Could you check a few things on this model? Use its own coordinates, in mm. Face numbers are marked on the shaded views. A direction names the side the tool comes from. Give positions to 0.01 mm unless a question says otherwise; leave off trailing zeros. Write each loop counter-clockwise with the first axis right and the second up, starting at its lowest first coordinate (ties: lowest second). Pieces come first, ordered by that corner, then holes. Notation, with made-up numbers: (-29.5, -13.75) - (6.5, -13.75) arc R22 ccw to (6.5, 3.25) - close; hole circle Ø5 at (61.5, 26.5). An arc over 180 degrees is marked (long way). Answer in a Markdown table with one row per item.
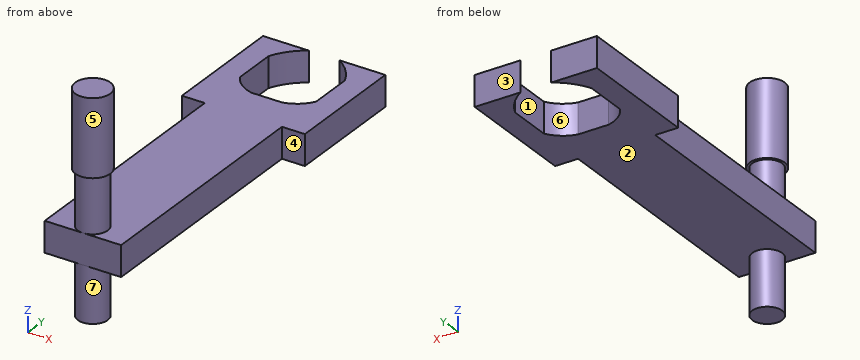
Autodesk Inventor part; units mm, degrees
ref_plane "YZ Plane" through (0, 0, 0) normal (1, 0, 0) x (0, 1, 0)
ref_plane "XZ Plane" through (0, 0, 0) normal (0, 1, 0) x (-1, 0, 0)
ref_plane "XY Plane" through (0, 0, 0) normal (0, 0, 1) x (1, 0, 0)
sketch "Sketch1" plane through (0, 0, 0) normal (0, 1, 0) x (-1, 0, 0)
  line L0 (0, 0) -> (0, -10)
  line L1 (0, 0) -> (25, 0)
  line L2 (25, 0) -> (25, -10)
  line L3 (25, -10) -> (0, -10)
  dimension "d0" = 10
  dimension "d1" = 25
  dimension "d2" = 10
extrude "Extrusion1" add sketch "Sketch1" along normal blind 120
sketch "Sketch2" plane through (-25, 0, 0) normal (0, 0, 1) x (1, 0, 0)
  line L0 (25, 0) -> (0, 0)
  line L1 (12.5, 0) -> (17.5, 0)
  line L2 (17.5, 0) -> (12.5, 0)
  line L3 (12.5, 0) -> (12.5, 4.9)
  circle A0 centre (12.5, 4.9) radius 4.9
  dimension "d5" = 5
  dimension "d6" = 4.9
extrude "Extrusion2" add sketch "Sketch2" along normal blind 18
sketch "Sketch3" plane through (-25, 120, 0) normal (0, 0, 1) x (1, 0, 0)
  line L0 (12.5, -120) -> (20.5, -120)
  line L1 (12.5, -120) -> (25, -120)
  dimension "d9" = 8
sketch "Sketch4" plane through (0, 0, 0) normal (1, 0, 0) x (0, 0, -1)
  point P0 (0, 0)
sketch "Sketch5" plane through (0, 0, 0) normal (1, 0, 0) x (0, 0, -1)
  point P0 (0, 0)
sketch "Sketch6" plane through (0, 0, 0) normal (1, 0, 0) x (0, 0, -1)
  point P0 (0, 0)
sketch "Sketch7" plane through (0, 0, 0) normal (1, 0, 0) x (0, 0, -1)
  point P0 (0, 0)
sketch "Sketch8" plane through (0, 0, -10) normal (0, 0, -1) x (-1, 0, 0)
  circle A0 centre (12.5, 4.9) radius 4.9
  circle A1 centre (12.5, 4.9) radius 4.9
  point P0 (0, 0)
  point P1 (12.5, 0)
extrude "Extrusion3" add sketch "Sketch8" along normal blind 18
sketch "Sketch9" plane through (-12.5, 4.9, 18) normal (0, 0, 1) x (1, 0, 0)
  circle A0 centre (0, 0) radius 5.75
  point P0 (12.5, -4.9)
  dimension "d12" = 11.5
extrude "Extrusion4" add sketch "Sketch9" along normal blind 25
sketch "Sketch10" plane through (-25, 120, 0) normal (0, 0, 1) x (1, 0, 0)
  line L0 (0, 0) -> (25, 0)
  line L1 (12.5, 0) -> (12.5, -28.5)
  line L2 (12.5, -28.5) -> (-0.5, -28.5)
  line L3 (-0.5, -28.5) -> (12.5, -28.5)
  line L4 (12.5, -28.5) -> (25.5, -28.5)
  line L5 (25.5, -28.5) -> (25.5, 0)
  line L6 (25.5, 0) -> (-0.5, 0)
  line L7 (-0.5, 0) -> (-0.5, -28.5)
  line L8 (12.5, 0) -> (7.5, 0)
  line L9 (7.5, 0) -> (17.5, 0)
  line L10 (25.5, 0) -> (25.5, -10)
  line L11 (25.5, -10) -> (25.5, -22)
  line L12 (-0.5, 0) -> (-0.5, -10)
  line L13 (-0.5, -10) -> (-0.5, -22)
  arc A0 (7.5, 0) -> (-0.5, -22) centre (17.25, -16) ccw
  arc A1 (-0.5, -22) -> (12.5, -28.5) centre (10, -17.25) ccw
  line L14 (7.5, 0) -> (12.5, 0)
  arc A2 (25.5, -22) -> (17.5, 0) centre (7.75, -16) ccw
  arc A3 (12.5, -28.5) -> (25.5, -22) centre (15, -17.25) ccw
  line L15 (7.5, 0) -> (-7.5, 0)
  line L16 (-7.5, 0) -> (-7.5, -34)
  line L17 (-7.5, -34) -> (25, -34)
  line L18 (25, -120) -> (25, 0)
  line L19 (25, -34) -> (32.5, -34)
  line L20 (32.5, 0) -> (25, 0)
  line L21 (25, 0) -> (17.5, 0)
  line L22 (17.5, 0) -> (32.5, 0)
  line L23 (32.5, 0) -> (32.5, -34)
  point P0 (7.5, -28.5)
  point P1 (17.5, -28.5)
  point P2 (25, -22.9782)
  point P3 (25, -8.6856)
  dimension "d15" = 28.5
  dimension "d16" = 13
  dimension "d17" = 13
  dimension "d18" = 13
  dimension "d19" = 5
  dimension "d20" = 10
  dimension "d21" = 10
  dimension "d22" = 12
  dimension "d23" = 10
  dimension "d24" = 12
  dimension "d25" = 15
  dimension "d26" = 34
  dimension "d28" = 15
extrude "Extrusion5" cut sketch "Sketch10" against normal blind 10 contours L0 L1 L2 A1 L7 A0 | L0 A2 L18 A3 L4 L1
sketch "Sketch11" plane through (-25, 0, 0) normal (0, 0, 1) x (1, 0, 0)
  point P0 (25, 0)
sketch "Sketch12" plane through (-7.5, 120, 0) normal (0, 0, 1) x (1, 0, 0)
  line L0 (7.5, 0) -> (0, 0)
  line L1 (0, 0) -> (15, 0)
  line L2 (15, 0) -> (15, -40)
  line L3 (15, -40) -> (7.5, -40)
  line L4 (7.5, -120) -> (7.5, -22.9782)
  line L5 (7.5, -8.6856) -> (7.5, 0)
  line L6 (7.5, -40) -> (7.5, 0)
  line L7 (-10, 0) -> (-17.5, 0)
  line L8 (7.5, 0) -> (-17.5, 0)
  line L9 (-10, 0) -> (-25, 0)
  line L10 (-25, 0) -> (-25, -40.3744)
  line L11 (-25, -40.3744) -> (-17.5, -40.3744)
  line L12 (-17.5, -120) -> (-17.5, -22.9782)
  line L13 (-17.5, -8.6856) -> (-17.5, 0)
  line L14 (-17.5, -40.3744) -> (-17.5, 0)
  dimension "d31" = 15
  dimension "d32" = 40
  dimension "d33" = 15
extrude "Extrusion6" add sketch "Sketch12" against normal blind 10
ref_plane "Work Plane1" through (-12.5, 0, 0) normal (1, 0, 0) x (0, 0, -1)
properties part number "brazo2"
1) We'd pull the mould along Y, two halves only. Please class the marked faces 1, 2 and 3: +Y half, -Y half, draft (parallel to the pull), parting line (faces both ways), or undercut.
Check values:
| item | result |
|---|---|
| face 1 | undercut |
| face 2 | draft |
| face 3 | +Y half |
2) Imagine slicing it at B-B (y = 4.9). List the corners of the cut face in (x, z) for me.
Check values:
| item | result |
|---|---|
| outline | (-25, -10) - (-17.4, -10) - (-17.4, -28) - (-7.6, -28) - (-7.6, -10) - (0, -10) - (0, 0) - (-7.6, 0) - (-7.6, 18) - (-6.75, 18) - (-6.75, 43) - (-18.25, 43) - (-18.25, 18) - (-17.4, 18) - (-17.4, 0) - (-25, 0) - close |
3) Imagine slicing it at D-D (x = 5.5). List the corners of the cut face in (y, z) for me, then the cut area to 3 significant figures.
Check values:
| item | result |
|---|---|
| outline | (80, -10) - (120, -10) - (120, 0) - (80, 0) - close |
| area | 400 mm2 |
4) Imagine slicing it at C-C (z = 2). List the corners of the cut face in (x, y) for me.
Check values:
| item | result |
|---|---|
| outline | circle Ø9.8 at (-12.5, 4.9) |
5) Will these pins go through, and if not, where does the flat tip stop? P1, Ø12, axis at x = -28.5, y = 52.5, coming from the -Z side; P2, Ø6, axis at x = -7, z = -11, coming from the -Y side; P3, Ø6, axis at y = 37.5, z = -12, coming from the -X side.
Check values:
| item | result |
|---|---|
| P1 | stops at z = -10 |
| P2 | stops at y = 0 |
| P3 | stops at x = -25 |
6) Imagine slicing it at A-A (x = -20). List the corners of the cut face in (y, z) for me.
Check values:
| item | result |
|---|---|
| outline | (0, -10) - (92.37, -10) - (92.37, 0) - (0, 0) - close; (118.18, -10) - (120, -10) - (120, 0) - (118.18, 0) - close |
7) On a 3-axis mill with a long thin cutter (end or side, diameter ignored), from which of +Z, -Z, +X, -X, +Y, -Y can I reach the whole of each face in a straight line? I mean the marked faces 4, 5, 6 and 7. Say none if no direction works.
Check values:
| item | result |
|---|---|
| face 4 | +Z, -Z, +X, -Y |
| face 5 | +Z |
| face 6 | +Z, -Z |
| face 7 | -Z |
8) If I drill on line 1 (Y direction, x = -13, z = -21); line 2 (Z direction, x = -29, y = 82); line 3 (Y direction, x = -5.5, z = -9.5), over which ranges is the centre line in solid material (lowest first)?
Check values:
| item | result |
|---|---|
| line 1 | y = 0.03 to 9.77 |
| line 2 | z = -10 to 0 |
| line 3 | y = 0 to 92.14, 118.59 to 120 |
